Part model, mm, in its own coordinate system. Face numbers are marked on the shaded views. A direction names the side the tool comes from. Give positions to 0.01 mm unless a question says otherwise; leave off trailing zeros. Order: outer loops, then holes, each group sorted by start corner. A loop starts at its lowest first (then second) coordinate and runs counter-clockwise, first axis right, second up.
1. Slice it at A-A on z = 34. List the corners of the cut face in (x, y).
2. Slice it at C-C on x = 0. List the corners of the cut face in (y, z), and give its area (3 significant figures).
3. Which spindle directions (+Z, -Z, +X, -X, +Y, -Y) get a long thin tool onto all of the face, cutting with end or side? Do the marked faces 4, 5 and 6. Say none if no direction does.
4. Slice it at D-D on x = 45. List the corners of the cut face in (y, z).
5. Mould opens along Y. For the marked faces 1, 2 and 3 say: +Y half, -Y half, draft (parallel to the pull), parting line (faces both ways), or undercut.
6. Drop flat-ended pins along their axis: pin 1 Ø22.5 at (x, y) = (-7, -0.5) entering from +Z; pin 2 Ø8 at (x, z) = (-4.5, -10) entering from +Y; pin 3 Ø2 at (x, y) = (-26.5, 35) entering from +Z. Give the stop position or say it passes through.
7. Slice it at B-B on y = 75. List the corners of the cut face in (x, z).
8. Probe line 1 (Y direction, x = 0, z = 45.5); line 2 (Y direction, x = 0, z = 52); line 3 (X direction, y = -75, z = 45). List the from-to ranges inside material, lowest first.
from build123d import *

# Parameters (mm, degrees)
SKETCH1_R           = 15
BOSS_EXTRUDE1_DEPTH = 100
BOSS_EXTRUDE2_START = -50
SKETCH2_W           = 115
SKETCH2_H           = 30
BOSS_EXTRUDE2_DEPTH = 105
FILLET1_R           = 20
SKETCH3_W           = 80
SKETCH3_H           = 45
BOSS_EXTRUDE3_DEPTH = 8
CUT_EXTRUDE1_DEPTH  = 268.5


with BuildPart() as part:
    # Sketch1 → Boss-Extrude1 (new body)
    with BuildSketch(Plane.XY):
        with BuildLine():
            Line((-40, 102.46950766), (-40, -102.46950766))
            ThreePointArc((-40, -102.46950766), (-36.757315886, -103.676900652), (-33.47826087, -104.781706653))
            ThreePointArc((-33.47826087, -104.781706653), (-30.962135735, -106.595672378), (-30, -109.544511501))
            Line((-30, -109.544511501), (-30, -165))
            Line((-30, -165), (30, -165))
            Line((30, -165), (30, -109.544511501))
            ThreePointArc((30, -109.544511501), (30.962135735, -106.595672378), (33.47826087, -104.781706653))
            ThreePointArc((33.47826087, -104.781706653), (36.757315886, -103.676900652), (40, -102.46950766))
            Line((40, -102.46950766), (40, 102.46950766))
            ThreePointArc((40, 102.46950766), (0, 110), (-40, 102.46950766))
        make_face()
        with Locations((0, 75)):
            Circle(SKETCH1_R, mode=Mode.SUBTRACT)
        with Locations(Location((0, -75, 0), (0, 0, 180))):
            Circle(SKETCH1_R, mode=Mode.SUBTRACT)
    extrude(amount=BOSS_EXTRUDE1_DEPTH)

    # Sketch2 → Boss-Extrude2 (add, symmetric)
    with BuildSketch(Plane.XY.offset(100).offset(BOSS_EXTRUDE2_START)):
        with Locations((0, -180)):
            Rectangle(SKETCH2_W, SKETCH2_H)
    extrude(amount=BOSS_EXTRUDE2_DEPTH, both=True)

    # Fillet1
    fillet1_edges = [part.edges().sort_by_distance(p)[0] for p in [
        (0, -165, 0),
        (0, -165, 100),
        (30, -165, 50),
        (-30, -165, 50),
    ]]
    fillet(fillet1_edges, radius=FILLET1_R)

    # Sketch3 → Boss-Extrude3 (add)
    with BuildSketch(Plane.XY.offset(100)):
        Rectangle(SKETCH3_W, SKETCH3_H)
    extrude(amount=BOSS_EXTRUDE3_DEPTH)

    # Sketch4 → Cut-Extrude1 (cut, through all)
    with BuildSketch(Plane.ZY.offset(40)):
        with BuildLine():
            Line((-70, -40), (50, -40))
            ThreePointArc((50, -40), (90, 0), (50, 40))
            Line((50, 40), (-70, 40))
            Line((-70, 40), (-70, -40))
        make_face()
    extrude(amount=-CUT_EXTRUDE1_DEPTH, mode=Mode.SUBTRACT)


solid = part.part
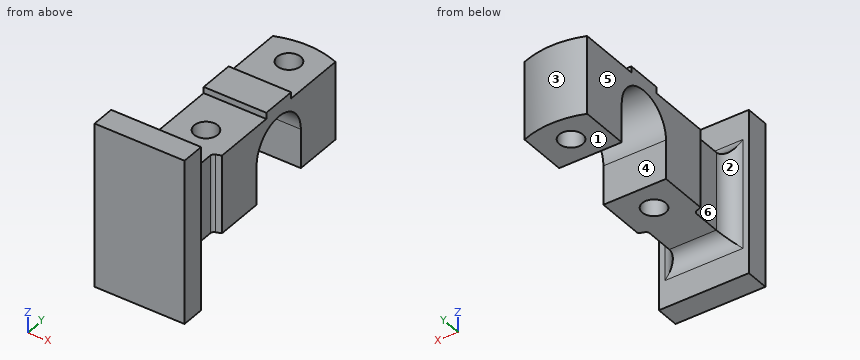
Data:
1. outline: (-57.5, -195) - (57.5, -195) - (57.5, -165) - (50, -165) arc R20 cw to (30, -145) - (30, -109.54) arc R5 cw to (33.48, -104.78) arc R110 ccw to (40, -102.47) - (40, -40) - (-40, -40) - (-40, -102.47) arc R110 ccw to (-33.48, -104.78) arc R5 cw to (-30, -109.54) - (-30, -145) arc R20 cw to (-50, -165) - (-57.5, -165) - close; (-40, 40) - (40, 40) - (40, 102.47) arc R110 ccw to (-40, 102.47) - close; hole circle Ø30 at (0, -75); hole circle Ø30 at (0, 75)
2. outline: (-195, -55) - (-165, -55) - (-165, -20) arc R20 cw to (-145, 0) - (-90, 0) - (-90, 100) - (-145, 100) arc R20 cw to (-165, 120) - (-165, 155) - (-195, 155) - close; (-60, 0) - (-40, 0) - (-40, 50) arc R40 cw to (40, 50) - (40, 0) - (60, 0) - (60, 100) - (22.5, 100) - (22.5, 108) - (-22.5, 108) - (-22.5, 100) - (-60, 100) - close; (90, 0) - (110, 0) - (110, 100) - (90, 100) - close
2. area: 21,800 mm2
3. face 4: -Z, +X, -X
3. face 5: +Z, -Z, -X, +Y
3. face 6: +Z, -Z, -X
4. outline: (-195, -55) - (-165, -55) - (-165, -20) arc R20 cw to (-164.36, -15) - (-164.36, 115) arc R20 cw to (-165, 120) - (-165, 155) - (-195, 155) - close
5. face 1: draft
5. face 2: undercut
5. face 3: +Y half
6. pin 1: stops at z = 108
6. pin 2: stops at y = -159.28
6. pin 3: stops at z = 100
7. outline: (-40, 0) - (-15, 0) - (-15, 100) - (-40, 100) - close; (15, 0) - (40, 0) - (40, 100) - (15, 100) - close
8. line 1: y = -195 to -90, -60 to -40, 40 to 60, 90 to 110
8. line 2: y = -195 to -90, -60 to -39.95, 39.95 to 60, 90 to 110
8. line 3: x = -40 to -15, 15 to 40
